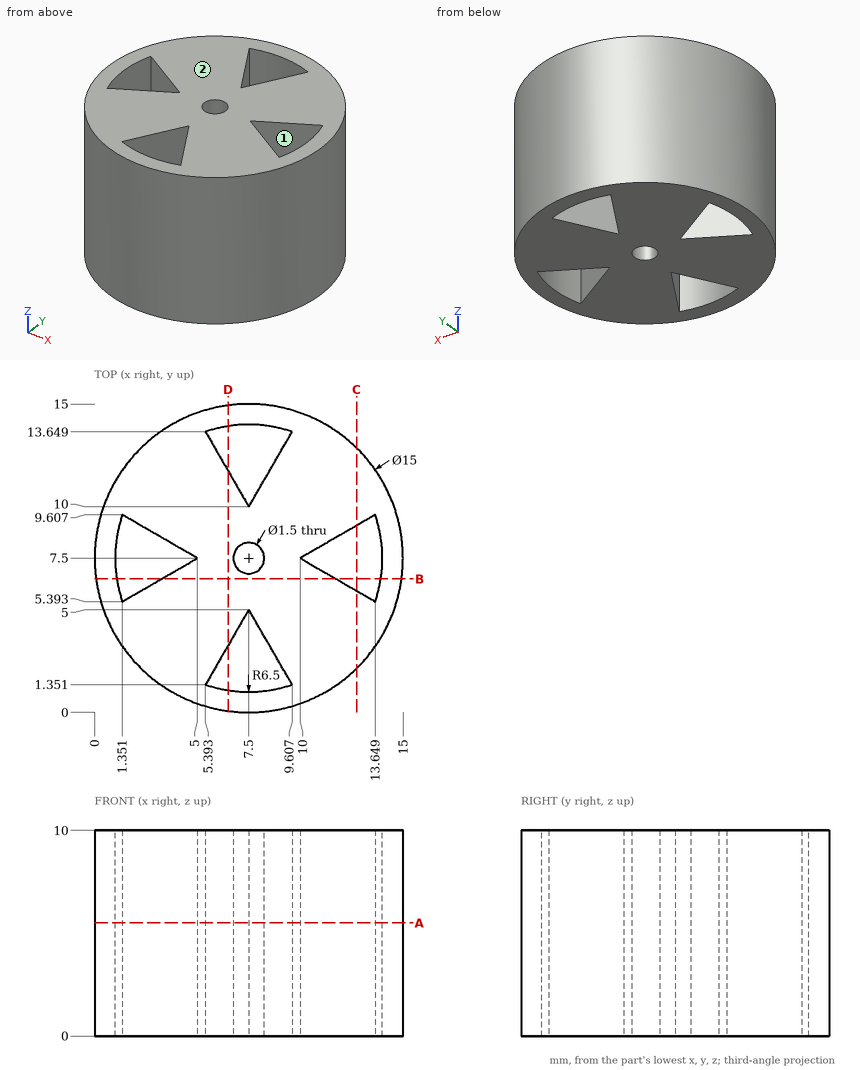
Geometry check sheet. Reference: drawing and pictorial views, mm from the part's lowest x, y, z. A direction names the side the tool comes from. Give positions to 0.01 mm unless a question says otherwise; leave off trailing zeros. Write each loop counter-clockwise with the first axis right and the second up, starting at its lowest first coordinate (ties: lowest second). Pieces come first, ordered by that corner, then holes. Notation, with made-up numbers: (68.25, 82) -> (81.25, 82) arc R19 cw to (81.25, 92) -> close; hole circle Ø9 at (-11, 32). An arc over 180 degrees is marked (long way). One line per item, written item: value. Start each with the question number.
Item 1: Section check B-B on y = 6.5. Record the cut outline in (x, z), then the cut area to 3 significant figures.
Item 2: Material ranges on probe 1 along Y at (x, z) = (9.25, 7.5); probe 2 along X at (y, z) = (8.75, 1.5) (1 decimal); probe 3 along X at (y, z) = (5.5, 1) (1 decimal), recorded low to high. Write a range as from..to.
Item 3: Gauge pin test, flat ends, axial feed: pin 1 (1 mm diameter, centred on y = 5.5, z = 3.5, fed in from +X); pin 2 (3 mm diameter, centred on y = 3.5, z = 5.5, fed in from +X); pin 3 (3 mm diameter, centred on y = 3, z = 6.5, fed in from +X); pin 4 (2.5 mm diameter, centred on x = 7.5, y = 7.5, fed in from -Z). Record the tip position at first contact, or that the pin passes through.
Item 4: Tool access check on the marked faces 1 and 2. Record the directions out of +Z, -Z, +X, -X, +Y, -Y that give a thin tool (end or side, any length) a straight path to the whole face; none if there is none.
Item 5: Section check A-A on z = 5.5. Record the cut outline in (x, y).
Item 6: Section check C-C on x = 12.75. Record the cut outline in (y, z).
Results list:
1. outline: (0.07, 0) -> (1.08, 0) -> (1.08, 10) -> (0.07, 10) -> close; (3.27, 0) -> (11.73, 0) -> (11.73, 10) -> (3.27, 10) -> close; (13.92, 0) -> (14.93, 0) -> (14.93, 10) -> (13.92, 10) -> close
1. area: 105 mm²
2. probe 1: 0.21..1.24, 1.97..13.03, 13.76..14.79
2. probe 2: 0.1..1.1, 2.8..12.2, 13.9..14.9
2. probe 3: 0.3..1.3, 1.5..13.5, 13.7..14.7
3. pin 1: x = 14.85
3. pin 2: x = 14.57
3. pin 3: x = 14.37
3. pin 4: z = 0
4. face 1: +Z, -Z
4. face 2: +Z, +X, -X, +Y, -Y
5. outline: circle Ø15 at (7.5, 7.5); hole (1.35, 5.39) -> (5, 7.5) -> (1.35, 9.61) arc R6.5 ccw to start; hole (5.39, 1.35) arc R6.5 ccw to (9.61, 1.35) -> (7.5, 5) -> close; hole (5.39, 13.65) -> (7.5, 10) -> (9.61, 13.65) arc R6.5 ccw to start; hole circle Ø1.5 at (7.5, 7.5); hole (10, 7.5) -> (13.65, 5.39) arc R6.5 ccw to (13.65, 9.61) -> close
6. outline: (2.14, 0) -> (5.91, 0) -> (5.91, 10) -> (2.14, 10) -> close; (9.09, 0) -> (12.86, 0) -> (12.86, 10) -> (9.09, 10) -> close
